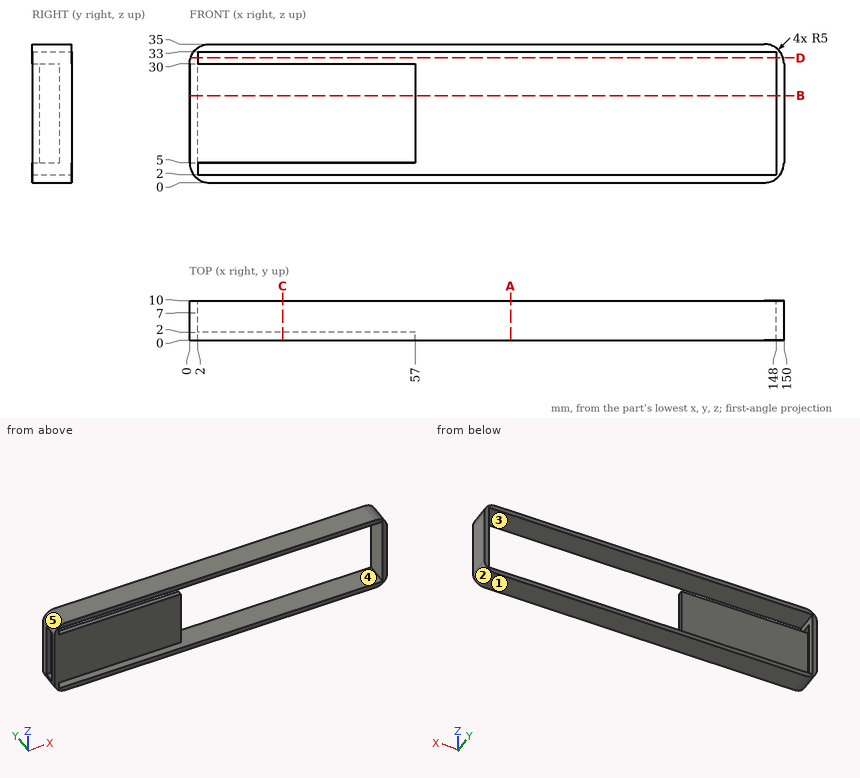
The figure shows three views and two pictorial views of one solid part (mm, origin at its lowest corner). Answer the questions. A direction names the side the tool comes from. Round coordinates to 2 decimals unless told otherwise and drop trailing zeros. Write each loop counter-clockwise with the first axis right and the second up, starting at its lowest first coordinate (ties: lowest second). Pieces come first, ordered by that corner, then holes. Notation, with made-up numbers: M 23,51 L 50,51 A6 cw 50,56 Z; hole C 88.5,79.25 d3. An arc over 180 degrees is marked long. Use a Markdown table: item, result.
1) The part is cut by section C-C on x = 23.5. Give the vertices of the cut face in (y, z), plus the area to 3 significant figures.
Taken from the geometry:
| item | result |
|---|---|
| outline | M 0,0 L 10,0 L 10,2 L 0,2 Z; M 0,5 L 2,5 L 2,30 L 0,30 Z; M 0,33 L 10,33 L 10,35 L 0,35 Z |
| area | 90.0 mm2 |
2) Flat-ended cylindrical pins translate along their axes: pin 1 (2 mm diameter, centred on x = 1, y = 5.5, fed in from +Z); pin 2 (12.5 mm diameter, centred on x = 39, z = 23, fed in from +Y); pin 3 (2 mm diameter, centred on x = 59, z = 22.5, fed in from +Y); pin 4 (1 mm diameter, centred on x = 1, y = 4.5, fed in from -Z). Find the tip coordinate at first contact, or state that the pin passes through.
Taken from the geometry:
| item | result |
|---|---|
| pin 1 | stops at z = 34 |
| pin 2 | stops at y = 2 |
| pin 3 | passes through |
| pin 4 | stops at z = 1.43 |
3) The part is cut by section B-B on z = 22. Give the vertices of the cut face in (x, y).
Taken from the geometry:
| item | result |
|---|---|
| outline | M 0,0 L 57,0 L 57,2 L 0,2 Z; M 0,7 L 2,7 L 2,10 L 0,10 Z; M 148,0 L 150,0 L 150,10 L 148,10 Z |
4) Consider line 1 (Z direction, x = 21, y = 0.75); line 2 (Z direction, x = 46, y = 5.25); line 3 (X direction, y = 1.75, z = 9). Determine where each line is inside the solid, lowest interval first. Write a range as [from, to].
Taken from the geometry:
| item | result |
|---|---|
| line 1 | z = [0, 2], [5, 30], [33, 35] |
| line 2 | z = [0, 2], [33, 35] |
| line 3 | x = [0, 57], [148, 150] |
5) Determine the mould class of the marked faces 1, 2 and 3 for opening direction X: pulls with the +X half, pulls with the -X half, needs draft (parallel to the pull), parting line crosses it, or undercut.
Taken from the geometry:
| item | result |
|---|---|
| face 1 | needs draft |
| face 2 | pulls with the +X half |
| face 3 | undercut |
6) The part is cut by section A-A on x = 81. Give the vertices of the cut face in (y, z), plus the area to 3 significant figures.
Taken from the geometry:
| item | result |
|---|---|
| outline | M 0,0 L 10,0 L 10,2 L 0,2 Z; M 0,33 L 10,33 L 10,35 L 0,35 Z |
| area | 40.0 mm2 |
7) Which of the six approach directions +Z, -Z, +X, -X, +Y, -Y give full straight-line access (tool end or side, diameter ignored) to the marked faces 4 and 5?
Taken from the geometry:
| item | result |
|---|---|
| face 4 | +Y, -Y |
| face 5 | +Z, -X, +Y, -Y |
8) The part is cut by section D-D on z = 31.5. Give the vertices of the cut face in (x, y).
Taken from the geometry:
| item | result |
|---|---|
| outline | M 0.23,0 L 2,0 L 2,10 L 0.23,10 Z; M 148,0 L 149.77,0 L 149.77,10 L 148,10 Z |
